The figure shows three views and two pictorial views of one solid part (mm, origin at its lowest corner). Answer the questions. A direction names the side the tool comes from. Give positions to 0.01 mm unless a question says otherwise; leave off trailing zeros. Loops run counter-clockwise (first coordinate to the right, second up) from the corner with the lowest first, then second, coordinate; pieces in that order, holes last. Notation, with made-up numbers: (77.25, -39) -> (103.25, -39) arc R25 ccw to (103.25, -27) -> close; hole circle Ø8 at (65.25, 41). An arc over 180 degrees is marked (long way). Answer as CSV lines item,"result". Start each with the question number.
1. Determine the mould class of the marked faces 1, 2 and 3 for opening direction X: +X half, -X half, draft (parallel to the pull), parting line (faces both ways), or undercut.
2. Find the intervals of material crossed by line 1 along Z through (x, y) = (57.5, 22); line 2 along Y through (x, z) = (40, 14.25) (1 decimal); line 3 along Y through (x, z) = (27, 14.5), in increasing order.
3. A tool of negligible diameter and unlimited length cuts with its end or side. For the marked faces 4 and 5, from which of +Z, -Z, +X, -X, +Y, -Y can it reach the whole face along a straight path? Write none if from no direction.
4. Find section C-C, the plane z = 11.75. Give the vertices of the cut face in (x, y).
5. Flat-ended cylindrical pins translate along their axes: pin 1 Ø6 at (x, z) = (47, 5.5) entering from -Y; pin 2 Ø8 at (y, z) = (37.5, 19) entering from -X; pin 3 Ø1 at (x, y) = (42, 41.5) entering from +Z; pin 4 Ø8 at (x, z) = (54.5, 15) entering from -Y. Find the tip coordinate at first contact, or state that the pin passes through.
6. Find section A-A, the plane y = 33. Give the vertices of the cut face in (x, z).
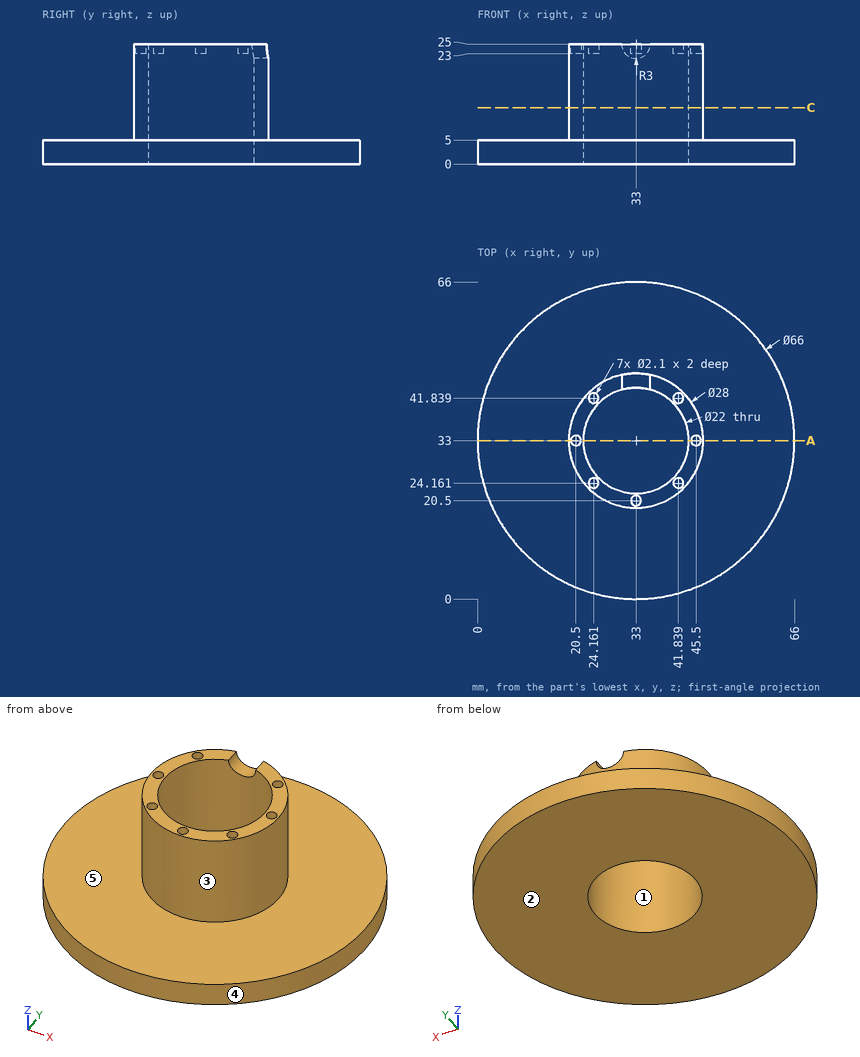
Resolved:
1,face 1,"undercut"
1,face 2,"draft"
1,face 3,"parting line"
2,line 1,"z = 0 to 5"
2,line 2,"y = 20.9 to 24.5, 41.5 to 45.1"
2,line 3,"y = 20.35 to 23.78, 42.22 to 45.65"
3,face 4,"+Z, -Z"
3,face 5,"+Z"
4,outline,"circle Ø28 at (33, 33); hole circle Ø22 at (33, 33)"
5,pin 1,"stops at y = 1.9"
5,pin 2,"stops at x = 19.01"
5,pin 3,"stops at z = 23"
5,pin 4,"passes through"
6,outline,"(0, 0) -> (22, 0) -> (22, 25) -> (21.55, 25) -> (21.55, 23) -> (19.45, 23) -> (19.45, 25) -> (19, 25) -> (19, 5) -> (0, 5) -> close; (44, 0) -> (66, 0) -> (66, 5) -> (47, 5) -> (47, 25) -> (46.55, 25) -> (46.55, 23) -> (44.45, 23) -> (44.45, 25) -> (44, 25) -> close"
